Can you work these out from the model? Positions are in its coordinate system, mm. Face numbers are marked on the shaded views. A direction names the side the tool comes from. Give positions to 0.01 mm unless a question says otherwise; leave off trailing zeros. Loops run counter-clockwise (first coordinate to the right, second up) from the corner with the lowest first, then second, coordinate; pieces in that order, holes last. Notation, with made-up numbers: M -35.75,77 L -19.75,77 A23 ccw -19.75,113 Z; hole C 39.25,74.5 d10. An arc over 180 degrees is marked long. Use CSV: the item, a comma, the result in double quotes.
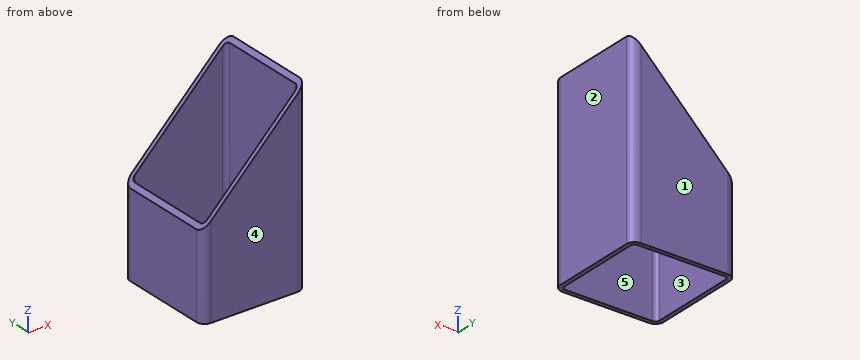
Autodesk Inventor part; units mm, degrees
ref_plane "Start Plane" through (0, 0, 25) normal (0, 0, 1) x (1, 0, 0)
ref_plane "End Plane" through (0, 0, 115.5) normal (0, 0, 1) x (1, 0, 0)
ref_plane "Work Plane4" through (25, 0, 115.5) normal (-0.7071, 0, 0.7071) x (0.7071, 0, 0.7071)
ref_plane "Start Plane" through (0, 0, 25) normal (0, 0, 1) x (1, 0, 0)
ref_plane "End Plane" through (0, 0, 115.5) normal (0, 0, 1) x (1, 0, 0)
sketch "Sketch" plane through (0, 0, 0) normal (0, 0, 1) x (1, 0, 0)
  line L0 (-25, -21) -> (-25, 21)
  line L1 (-21, 25) -> (21, 25)
  line L2 (25, 21) -> (25, -21)
  line L3 (21, -25) -> (-21, -25)
  arc A0 (-25, -21) -> (-21, -25) centre (-21, -21) ccw
  arc A1 (25, 21) -> (21, 25) centre (21, 21) ccw
  arc A2 (-21, 25) -> (-25, 21) centre (-21, 21) ccw
  arc A3 (21, -25) -> (25, -21) centre (21, -21) ccw
  arc A4 (-21, 23) -> (-23, 21) centre (-21, 21) ccw
  line L4 (-21, 23) -> (21, 23)
  arc A5 (23, 21) -> (21, 23) centre (21, 21) ccw
  line L5 (23, 21) -> (23, -21)
  arc A6 (21, -23) -> (23, -21) centre (21, -21) ccw
  line L6 (21, -23) -> (-21, -23)
  arc A7 (-23, -21) -> (-21, -23) centre (-21, -21) ccw
  line L7 (-23, -21) -> (-23, 21)
  line L8 (0, 36.1598) -> (0, -36.1598) construction
  line L9 (-36.1598, 0) -> (36.1598, 0) construction
  dimension "d7" = 4
  dimension "d9" = 50
  dimension "d11" = 50
  dimension "d12" = 2
  dimension "d15" = 25
  dimension "d16" = 25
extrude "Body" add sketch "Sketch" along normal up to surface (90.5 mm away) from surface at 25
sketch "Sketch3" plane through (0, 0, 0) normal (0, 0, 1) x (1, 0, 0)
  line L0 (0, 0) -> (10, 0)
ref_plane "Work Plane3" through (0, 0, 0) normal (0, -1, 0) x (1, 0, 0)
sketch "Sketch4" plane through (0, 0, 0) normal (0, -1, 0) x (1, 0, 0)
  line L0 (-2, 25) -> (12, 25)
  line L1 (-2, 115.5) -> (12, 115.5)
  dimension "d18" = 90.5
ref_plane "Work Plane4" through (25, 0, 115.5) normal (-0.7071, 0, 0.7071) x (0.7071, 0, 0.7071)
split "Split1" plane through (25, 0, 115.5) removes the side toward (-0.7071, 0, 0.7071)
ref_plane "Work Plane5" through (21, -282.75, 25) normal (0, 0, -1) x (-1, 0, 0)
split "Split2" plane through (21, -282.75, 25) removes the side toward (0, 0, -1)
equation "\"d7\" = G_IR"
equation "\"d9\" = G_W"
equation "\"d11\" = G_H"
equation "\"d12\" = G_T"
equation "\"d15\" = 0.5 * d9"
equation "\"d16\" = 0.5 * d11"
equation "\"d3\" = G_L"
equation "\"G_W\" = 50"
equation "\"G_H\" = 50"
equation "\"G_T\" = 2"
equation "\"G_IR\" = 4"
equation "\"G_L\" = d18"
equation "\"G_OFFSET_START\" = -25"
equation "\"G_OFFSET_END\" = 25"
equation "\"d13\" = -G_OFFSET_START"
equation "\"d14\" = G_OFFSET_END + B_L"
equation "\"B_L\" = 90.5"
properties part number "ISO 10799-2 - 50x50x2 - 90.5" material "Steel, Galvanized"
Q1. I want a section at B-B, the plane y = 3. Please give me the cut outline in (x, z), then the cut area to 3 significant figures.
Model answer:
outline,"M -25,25 L -23,25 L -23,67.5 L -25,65.5 Z; M 23,25 L 25,25 L 25,115.5 L 23,113.5 Z"
area,"262 mm2"
Q2. I want a section at A-A, the plane x = 12. Please give me the cut outline in (y, z), then the cut area to 3 significant figures.
Model answer:
outline,"M -25,25 L -23,25 L -23,102.5 L -25,102.5 Z; M 23,25 L 25,25 L 25,102.5 L 23,102.5 Z"
area,"310 mm2"
Q3. I want a section at D-D, the plane z = 85. Please give me the cut outline in (x, y), then the cut area to 3 significant figures.
Model answer:
outline,"M -5.5,-25 L 21,-25 A4 ccw 25,-21 L 25,21 A4 ccw 21,25 L -5.5,25 L -5.5,23 L 21,23 A2 cw 23,21 L 23,-21 A2 cw 21,-23 L -5.5,-23 Z"
area,"209 mm2"
Q4. For the marked faces 4 and 5, which set-ups out of +Z, -Z, +X, -X, +Y, -Y let a thin tool reach every point of the face, with its end or its side?
Model answer:
face 4,"+Z, -Z, +X, -X, -Y"
face 5,"+Z, -Z"
Q5. Please list where these lines run through material, in increasing order: L1, parallel to Y at x = -2, z = 35.5; L2, parallel to X at y = -18.5, z = 87.5. Write a range as from..to.
Model answer:
L1,"-25..-23, 23..25"
L2,"23..25"
Q6. If we mould it in two halves opening along X, with no side actions, what happens to the marked faces 1, 2 and 3? For each: released by +X, released by -X, zero draft, split by the parting line, or undercut.
Model answer:
face 1,"zero draft"
face 2,"released by +X"
face 3,"undercut"
Q7. I'm going to push a flat-ended pin straight in: P1, Ø12.5, axis at y = 4, z = 82.5, coming from the -X side. Where does the tip first touch, or does it pass through?
Model answer:
P1,"x = 23"
Q8. I want a section at C-C, the plane z = 41.5. Please give me the cut outline in (x, y).
Model answer:
outline,"M -25,-21 A4 ccw -21,-25 L 21,-25 A4 ccw 25,-21 L 25,21 A4 ccw 21,25 L -21,25 A4 ccw -25,21 Z; hole M -23,-21 A2 ccw -21,-23 L 21,-23 A2 ccw 23,-21 L 23,21 A2 ccw 21,23 L -21,23 A2 ccw -23,21 Z"
